from build123d import *

# Parameters (mm, degrees)
SKETCH_1_R      = 10.75
SKETCH_1_R_2    = 7.75
EXTRUDE_1_DEPTH = 620
SKETCH_2_R      = 15.301580628
EXTRUDE_2_DEPTH = 110


with BuildPart() as part:
    # Эскиз1 → Бобышка-Вытянуть1 (new body)
    with BuildSketch(Plane(origin=(0, 0, 0), x_dir=(1, 0, 0), z_dir=(0, 1, 0))):
        with Locations(Location((0, 0, 0), (0, 0, 270))):
            Circle(SKETCH_1_R)
        with Locations(Location((0, 0, 0), (0, 0, 270))):
            Circle(SKETCH_1_R_2, mode=Mode.SUBTRACT)
    extrude(amount=EXTRUDE_1_DEPTH)

    # Эскиз2 → Бобышка-Вытянуть2 (add)
    with BuildSketch(Plane(origin=(0, 620, 0), x_dir=(1, 0, 0), z_dir=(0, 1, 0))):
        with Locations(Location((0, 0, 0), (0, 0, 270))):
            Circle(SKETCH_2_R)
    extrude(amount=-EXTRUDE_2_DEPTH)


solid = part.part
Can you work these out from the model? Positions are in its coordinate system, mm. A direction names the side the tool comes from. Give positions to 0.01 mm unless a question says otherwise; leave off trailing zeros. Order: outer loops, then holes, each group sorted by start corner. A loop starts at its lowest first (then second) coordinate and runs counter-clockwise, first axis right, second up. Notation, with made-up numbers: (-19.5, 77.25) - (23.5, 77.25) arc R19 ccw to (23.5, 94.25) - close; hole circle Ø3 at (34, 2). An arc over 180 degrees is marked (long way). Write each question's results on one line, items separated by ' | '.
1) Suppose I cut it at C-C, the plane y = 81.5. Write out the boundary of the cut face in (x, z), then the cut area to 3 significant figures.
Final values:
outline: circle Ø21.5 at (0, 0); hole circle Ø15.5 at (0, 0) | area: 174 mm^2
2) Please list where these lines run through material, in increasing order: line 1 along X through (y, z) = (140, 0); line 2 along Y through (x, z) = (-10.5, 10.5). Write a range as [from, to].
Final values:
line 1: x = [-10.75, -7.75], [7.75, 10.75] | line 2: y = [510, 620]
3) If we mould it in two halves opening along Z, with no side actions, what happens to faces 3 (the face through (7.684, 251.43, -1.009)), 4 (the face through (7.27, 251.43, -7.92)), 5 (the face through (3.6, 510, -10.4))? For each: pulls with the +Z half, pulls with the -Z half, needs draft (parallel to the pull), parting line crosses it, or undercut.
Final values:
face 3: undercut | face 4: parting line crosses it | face 5: needs draft
4) On a 3-axis mill with a long thin cutter (end or side, diameter ignored), from which of +Z, -Z, +X, -X, +Y, -Y can I reach the whole of each face in a straight line? I mean faces 1 (the face through (0, 510, 0)), 2 (the face through (6, 0, 6)). Say none if no direction works.
Final values:
face 1: -Y | face 2: +Z, -Z, +X, -X, -Y
5) Suppose I cut it at B-B, the plane x = 0. Write out the boundary of the cut face in (y, z), then the cut area to 3 significant figures.
Final values:
outline: (0, -10.75) - (510, -10.75) - (510, -15.3) - (620, -15.3) - (620, 15.3) - (510, 15.3) - (510, 10.75) - (0, 10.75) - (0, 7.75) - (510, 7.75) - (510, -7.75) - (0, -7.75) - close | area: 6,430 mm^2
6) I'm going to push flat-ended pins straight in: pin 1 Ø3 at (x, y) = (-8.5, 65) entering from +Z; pin 2 Ø1 at (y, z) = (550.5, 3) entering from +X; pin 3 Ø5 at (x, z) = (4, 2.5) entering from -Y. Where does each tip first touch, or does it pass through?
Final values:
pin 1: stops at z = 8.16 | pin 2: stops at x = 15.1 | pin 3: stops at y = 510
7) Suppose I cut it at A-A, the plane z = 0. Write out the boundary of the cut face in (x, y).
Final values:
outline: (-15.3, 510) - (-10.75, 510) - (-10.75, 0) - (-7.75, 0) - (-7.75, 510) - (7.75, 510) - (7.75, 0) - (10.75, 0) - (10.75, 510) - (15.3, 510) - (15.3, 620) - (-15.3, 620) - close
